Source: CAD feature listing. Evaluate the final solid. Frame: model axes, mm. A direction names the side the tool comes from. Give positions to 0.01 mm unless a question says otherwise; leave off trailing zeros. Answer as a JSON object with one key per item and string values. Group by question number.
Item 1: Pull-direction query (X, two-part tool) for faces 4 (the face through (21, 18.6, -0.1)), 5 (the face through (19.27, 18.59, 1.13)), 6 (the face through (-15.418, 18.594, -0.273)), 7 (the face through (-21, 18.6, 0.1)); classes: pulls with the +X half, pulls with the -X half, needs draft (parallel to the pull), parting line crosses it, or undercut.
Item 2: First-contact query: pin 1 Ø12 at (x, y) = (-15, 27.5) entering from +Z. Flat tip, straight axial feed; report the tip coordinate or a pass-through.
Item 3: Access query for faces 1 (the face through (0.616, 9.367, -13.986)), 2 (the face through (0, 28, -6.5)), 3 (the face through (-2, 20.5, -6)). Directions: +Z, -Z, +X, -X, +Y, -Y. A direction counts if a zero-diameter tool reaches every point of the face in a straight line with its end or side. Return the directions, or none.
from build123d import *
from build123d.topology import SkipClean

# Parameters (mm, degrees)
CROQUIS1_R                   = 14
SALIENTE_EXTRUIR1_DEPTH      = 19
SALIENTE_EXTRUIR2_START      = -0.8
CROQUIS2_R                   = 2.1
SALIENTE_EXTRUIR2_DEPTH      = 0.8
SALIENTE_EXTRUIR3_REACH      = 51.591
SALIENTE_EXTRUIR3_END_RADIUS = 14
SALIENTE_EXTRUIR3_START      = 18
CROQUIS3_W                   = 12
CROQUIS3_H                   = 17.1
CROQUIS4_R                   = 4.5
SALIENTE_EXTRUIR4_DEPTH      = 1.5
CROQUIS5_R                   = 2.5
SALIENTE_EXTRUIR5_DEPTH      = 10
CROQUIS7_W                   = 6.557991655
CROQUIS7_H                   = 1.368399833
CROQUIS7_W_2                 = 6.403078466
CROQUIS7_H_2                 = 1.988052588
CORTAR_EXTRUIR1_DEPTH        = 6


with BuildPart() as part:
    # Croquis1 → Saliente-Extruir1 (new body)
    with BuildSketch(Plane(origin=(0, 0, 0), x_dir=(1, 0, 0), z_dir=(0, 1, 0))):
        with Locations(Location((0, 0, 0), (0, 0, 270))):
            Circle(CROQUIS1_R)
    extrude(amount=SALIENTE_EXTRUIR1_DEPTH)

    # Croquis2 → Saliente-Extruir2 (add)
    with SkipClean():  # the faces are left unmerged after this step: merging them gives an invalid solid
        with BuildSketch(Plane(origin=(0, 19, 0), x_dir=(1, 0, 0), z_dir=(0, 1, 0)).offset(SALIENTE_EXTRUIR2_START)):
            with BuildLine():
                Line((-17.5, 3.5), (-13.555441712, 3.5))
                ThreePointArc((-13.555441712, 3.5), (0, 14), (13.555441712, 3.5))
                Line((13.555441712, 3.5), (17.5, 3.5))
                ThreePointArc((17.5, 3.5), (21, 0), (17.5, -3.5))
                Line((17.5, -3.5), (13.555441712, -3.5))
                ThreePointArc((13.555441712, -3.5), (0, -14), (-13.555441712, -3.5))
                Line((-13.555441712, -3.5), (-17.5, -3.5))
                ThreePointArc((-17.5, -3.5), (-21, 0), (-17.5, 3.5))
            make_face()
            with Locations(Location((-17.5, 0, 0), (0, 0, 270))):
                Circle(CROQUIS2_R, mode=Mode.SUBTRACT)
            with Locations(Location((17.5, 0, 0), (0, 0, 270))):
                Circle(CROQUIS2_R, mode=Mode.SUBTRACT)
        extrude(amount=SALIENTE_EXTRUIR2_DEPTH)

    # Saliente-Extruir3: up to this cylinder (the profile starts outside it)
    with SkipClean():  # the faces are left unmerged after this step: merging them gives an invalid solid
        saliente_extruir3_end = Plane(origin=(0, 10.45, 0), z_dir=(0, -1, 0)) * Cylinder(SALIENTE_EXTRUIR3_END_RADIUS, 132.182, mode=Mode.PRIVATE)
        # Croquis3 → Saliente-Extruir3 (add, up to the surface)
        with BuildSketch(Plane.XY.offset(SALIENTE_EXTRUIR3_START), mode=Mode.PRIVATE) as saliente_extruir3_sk1:
            with Locations((0, 10.45)):
                Rectangle(CROQUIS3_W, CROQUIS3_H)
        saliente_extruir3_tool1 = extrude(saliente_extruir3_sk1.sketch, amount=-SALIENTE_EXTRUIR3_REACH, mode=Mode.PRIVATE) - saliente_extruir3_end
        add(saliente_extruir3_tool1.solids().sort_by_distance((0, 10.45, 18))[0])

    # Croquis4 → Saliente-Extruir4 (add)
    with SkipClean():  # the faces are left unmerged after this step: merging them gives an invalid solid
        with BuildSketch(Plane(origin=(0, 19, 0), x_dir=(1, 0, 0), z_dir=(0, 1, 0))):
            with Locations(Location((0, 8, 0), (0, 0, 270))):
                Circle(CROQUIS4_R)
        extrude(amount=SALIENTE_EXTRUIR4_DEPTH)

    # Croquis5 → Saliente-Extruir5 (add)
    with SkipClean():  # the faces are left unmerged after this step: merging them gives an invalid solid
        with BuildSketch(Plane(origin=(0, 20.5, 0), x_dir=(1, 0, 0), z_dir=(0, 1, 0))):
            with Locations(Location((0, 8, 0), (0, 0, 270))):
                Circle(CROQUIS5_R)
        extrude(amount=SALIENTE_EXTRUIR5_DEPTH)

    # Croquis7 → Cortar-Extruir1 (cut)
    with SkipClean():  # the faces are left unmerged after this step: merging them gives an invalid solid
        with BuildSketch(Plane(origin=(0, 30.5, 0), x_dir=(1, 0, 0), z_dir=(0, 1, 0))):
            with Locations((0.036072912, 10.184199917)):
                Rectangle(CROQUIS7_W, CROQUIS7_H)
            with Locations((-0.041383682, 5.505973706)):
                Rectangle(CROQUIS7_W_2, CROQUIS7_H_2)
        extrude(amount=-CORTAR_EXTRUIR1_DEPTH, mode=Mode.SUBTRACT)


solid = part.part
Worked answers:
{
 "1": {"face 4": "pulls with the +X half", "face 5": "undercut", "face 6": "undercut", "face 7": "pulls with the -X half"},
 "2": {"pin 1": "through"},
 "3": {"face 1": "-Y", "face 2": "+Z, +X, -X, +Y", "face 3": "+Y"}
}
